For this review, use the dimensioned drawing (mm, ordinates from the lowest corner) and the shaded views. A direction names the side the tool comes from. Round coordinates to 2 decimals unless told otherwise and drop trailing zeros. Write each loop counter-clockwise with the first axis right and the second up, starting at its lowest first coordinate (ties: lowest second). Pieces come first, ordered by that corner, then holes. Notation, with made-up numbers: M 15,48 L 24,48 A11 ccw 24,60 Z; hole C -18,40 d10. An arc over 180 degrees is marked long. One line per question, with ' | ' between items.
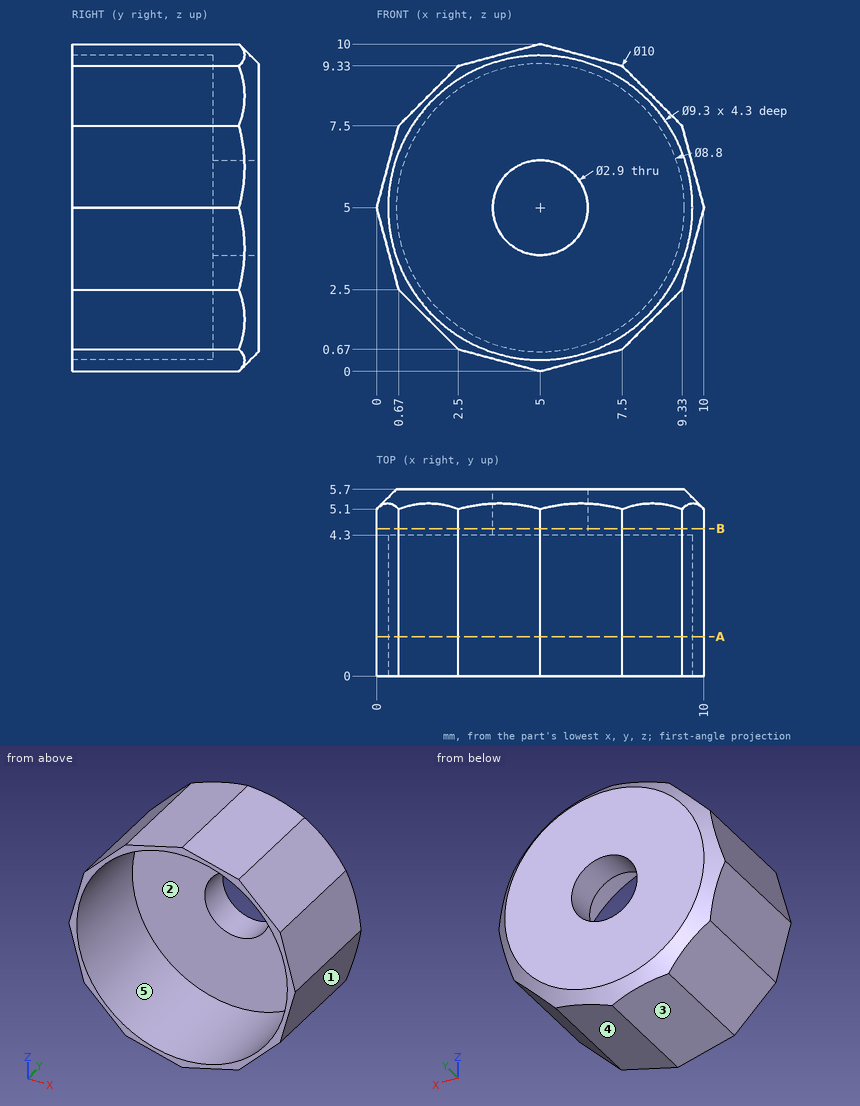
Item 1: Machinability: for the marked faces 1 and 2, which of the approach directions +Z, -Z, +X, -X, +Y, -Y give a long, thin tool a straight path to every point of the face, cutting with its end or side? Answer none if there is none.
Results:
face 1: -Z, +X, +Y, -Y | face 2: -Y
Item 2: To check wall thickness, follow line 1 along Y through (x, z) = (5.25, 7); line 2 along X through (y, z) = (4.4, 5.25); line 3 along Z through (x, y) = (5.75, 3.6). State the ranges of each line that lie inside material, in increasing order. Write a range as from..to.
Results:
line 1: 4.3..5.7 | line 2: 0.07..3.57, 6.43..9.93 | line 3: 0.2..0.41, 9.59..9.8
Item 3: Take a section at A-A (y = 1.2). Write out the cut boundary in (x, z).
Results:
outline: M 0,5 L 0.67,2.5 L 2.5,0.67 L 5,0 L 7.5,0.67 L 9.33,2.5 L 10,5 L 9.33,7.5 L 7.5,9.33 L 5,10 L 2.5,9.33 L 0.67,7.5 Z; hole C 5,5 d9.3
Item 4: Take a section at B-B (y = 4.5). Write out the cut boundary in (x, z), then the cut area to 3 significant figures.
Results:
outline: M 0,5 L 0.67,2.5 L 2.5,0.67 L 5,0 L 7.5,0.67 L 9.33,2.5 L 10,5 L 9.33,7.5 L 7.5,9.33 L 5,10 L 2.5,9.33 L 0.67,7.5 Z; hole C 5,5 d2.9 | area: 68.4 mm2
Item 5: Mouldability with a two-part tool opening along X and no side actions: class the marked faces 3, 4 and 5 as +X half, -X half, draft (parallel to the pull), parting line (faces both ways), or undercut.
Results:
face 3: -X half | face 4: +X half | face 5: undercut
